Can you work these out from the model? Positions are in its coordinate system, mm. Face numbers are marked on the shaded views. Coordinates: 2 decimals unless noted, no trailing zeros. Write each loop counter-clockwise with the first axis right and the second up, starting at its lowest first coordinate (ties: lowest second). Pieces come first, ordered by that corner, then holes. Notation, with made-up numbers: M -8,74 L 10,74 A29 cw 10,112 Z; hole C 4,-11.5 d5. An arc over 180 degrees is marked long. Use one line per item in the form item = value. Start each with the question number.
```python
from build123d import *

# Parameters (mm, degrees)
BOSS_EXTRUDE1_DEPTH = 30
INTERSECT1_START    = -64
INTERSECT1_DEPTH    = 64
HOLE1_D             = 10
HOLE1_CBORE_D       = 15
HOLE1_CBORE_DEPTH   = 10


with BuildPart() as part:
    # Sketch2 → Boss-Extrude1 (new body)
    with BuildSketch(Plane(origin=(0, 0, 0), x_dir=(1, 0, 0), z_dir=(0, 1, 0))):
        Polygon((0, 10), (0, 0), (0, -20), (-40, -45), (-55, -45), (-55, 10), align=None)
    extrude(amount=BOSS_EXTRUDE1_DEPTH)

    # Intersect1: read off the stored shape, not the designer's step
    # Intersect1 outline → Intersect1 (cut)
    with BuildSketch(Plane(origin=(0, 0, 0), x_dir=(0.5299989400031803, 0.8479983040050878, 0), z_dir=(0.8479983040050877, -0.5299989400031807, 0)).offset(INTERSECT1_START)):
        Polygon((-12.71997456, 45), (26.287947424, -1), (27, -1), (27, 45), align=None)
    extrude(amount=INTERSECT1_DEPTH, mode=Mode.SUBTRACT)

    # Hole1 (through all)
    with Locations(Plane.ZY.offset(55)):
        with Locations((0, 15)):
            CounterBoreHole(HOLE1_D / 2, HOLE1_CBORE_D / 2, HOLE1_CBORE_DEPTH)


solid = part.part
```
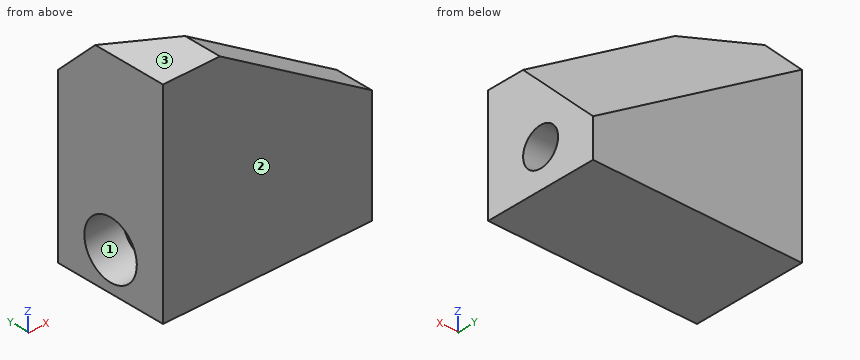
1) Suppose I cut it at C-C on x = -10. Please give me the cut outline in (y, z).
2) Suppose I cut it at B-B on z = 33.5. Please give me the cut outline in (x, y).
3) Please list where these lines run through material, in increasing order: line 1 (Y direction, x = -51.5, z = 0); line 2 (Y direction, x = -12, z = 0); line 3 (X direction, y = 24, z = 34.5).
4) If we mould it in two halves opening along Y, with no side actions, what happens to the marked faces 1, 2 and 3? For each: +Y half, -Y half, draft (parallel to the pull), parting line (faces both ways), or undercut.
5) Will these pins go through, and if not, where does the flat tip stop? pin 1 Ø4 at (x, y) = (-16.5, 4) entering from +Z; pin 2 Ø12 at (x, y) = (-7, 17) entering from +Z; pin 3 Ø3 at (x, y) = (-27, 24.5) entering from +Z.
6) Suppose I cut it at A-A on y = 15. Please give me the cut outline in (x, z), and give its area (4 significant figures).
7) Suppose I cut it at D-D on y = 4. Please give me the cut outline in (x, z).
Computed values:
q1.outline = M 0,-10 L 30,-10 L 30,6.25 L 10,26.25 L 0,26.25 Z; hole C 15,0 d10
q2.outline = M -55,0 L -21.6,0 L -21.6,10 L -53.6,30 L -55,30 Z
q3.line_1 = 0 to 7.5, 22.5 to 30
q3.line_2 = 0 to 10, 20 to 30
q3.line_3 = -55 to -45.6
q4.face_1 = undercut
q4.face_2 = -Y half
q4.face_3 = draft
q5.pin_1 = 31.56
q5.pin_2 = 24.45
q5.pin_3 = 24.14
q6.outline = M -55,-10 L 0,-10 L 0,-5 L -45,-5 L -45,-7.5 L -55,-7.5 Z; M -55,7.5 L -45,7.5 L -45,5 L 0,5 L 0,15 L -48,45 L -55,45 Z
q6.area = 1,705 mm²
q7.outline = M -55,-10 L 0,-10 L 0,20 L -40,45 L -55,45 Z
